Could you check a few things on this drawing? It's one solid part, dimensions in mm from its lowest x, y, z. Coordinates: 2 decimals unless noted, no trailing zeros. Loops run counter-clockwise (first coordinate to the right, second up) from the corner with the lowest first, then second, coordinate; pieces in that order, holes last. Notation, with made-up numbers: M 2.5,19.5 L 11.5,19.5 A19 ccw 11.5,47.5 Z; hole C -32,-23 d3. An arc over 180 degrees is marked long. Use one line per item in the form item = value. Start each with the question number.
(1) Please list where these lines run through material, in increasing order: L1, parallel to Y at x = 11, z = 2.4; L2, parallel to Y at x = 36, z = 1.5; L3, parallel to X at y = 30.5, z = 2.7.
(2) Imagine slicing it at A-A, the plane x = 36. Please give me the cut outline in (y, z) (1 decimal).
(3) Imagine slicing it at D-D, the plane y = 13. Please give me the cut outline in (x, z) (1 decimal).
(4) Imagine slicing it at B-B, the plane z = 1.35. Please give me the cut outline in (x, y), and give its area (3 significant figures).
(5) Imagine slicing it at C-C, the plane x = 11. Please give me the cut outline in (y, z) (1 decimal).
(6) Will these pins go through, and if not, where does the flat tip stop? P1, Ø1, axis at y = 8, z = 2.5, coming from the +X side; P2, Ø4, axis at x = 11, y = 55, coming from the +Z side; P3, Ø1, axis at y = 30.5, z = 1.5, coming from the +X side.
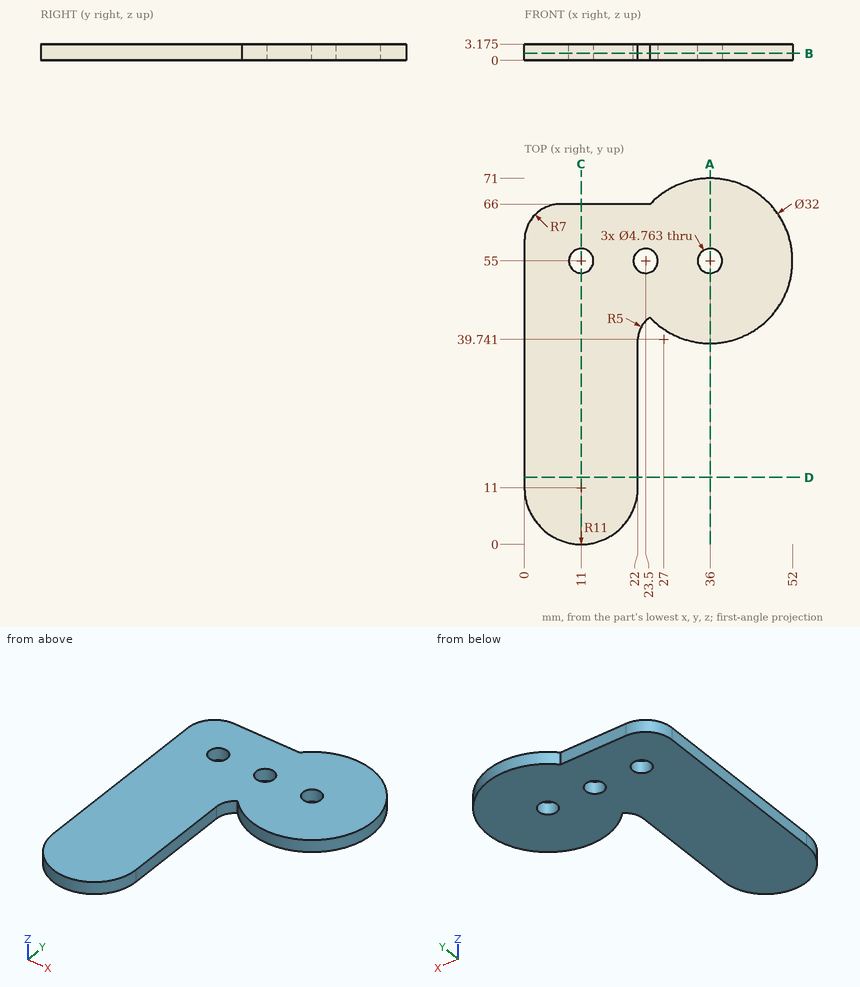
Answer:
q1.L1 = 0 to 52.62, 57.38 to 66
q1.L2 = 39 to 52.62, 57.38 to 71
q1.L3 = 0 to 22
q2.outline = M 39,0 L 52.6,0 L 52.6,3.2 L 39,3.2 Z; M 57.4,0 L 71,0 L 71,3.2 L 57.4,3.2 Z
q3.outline = M 0,0 L 22,0 L 22,3.2 L 0,3.2 Z
q4.outline = M 0,11 A11 ccw 22,11 L 22,39.74 A5 cw 24.38,44 A16 ccw long 24.38,66 L 7,66 A7 ccw 0,59 Z; hole C 11,55 d4.76; hole C 23.5,55 d4.76; hole C 36,55 d4.76
q4.area = 2,130 mm²
q5.outline = M 0,0 L 52.6,0 L 52.6,3.2 L 0,3.2 Z; M 57.4,0 L 66,0 L 66,3.2 L 57.4,3.2 Z
q6.P1 = 21.71
q6.P2 = through
q6.P3 = 22
